from build123d import *

# Parameters (mm, degrees)
ESBO_O1_R                = 3.5
ESBO_O1_R_2              = 3
ESBO_O1_R_3              = 1.6
RESSALTO_EXTRUS_O1_DEPTH = 6


with BuildPart() as part:
    # Esboço1 → Ressalto-extrusão1 (new body)
    with BuildSketch(Plane(origin=(0, 0, 0), x_dir=(1, 0, 0), z_dir=(0, 1, 0))):
        with BuildLine():
            Line((188.965018959, -38.648697641), (188.965018959, 28))
            ThreePointArc((188.965018959, 28), (185.450300333, 36.485281374), (176.965018959, 40))
            Line((176.965018959, 40), (-176.090826953, 40))
            ThreePointArc((-176.090826953, 40), (-184.576108327, 36.485281374), (-188.090826953, 28))
            Line((-188.090826953, 28), (-188.090826953, -38.648697641))
            ThreePointArc((-188.090826953, -38.648697641), (-184.576108327, -47.133979015), (-176.090826953, -50.648697641))
            Line((-176.090826953, -50.648697641), (176.965018959, -50.648697641))
            ThreePointArc((176.965018959, -50.648697641), (185.450300333, -47.133979015), (188.965018959, -38.648697641))
        make_face()
        with Locations(Location((-62.734509176, 0, 0), (0, 0, 90))):
            Circle(ESBO_O1_R, mode=Mode.SUBTRACT)
        with Locations(Location((176.748138959, -38.431817641, 0), (0, 0, 90))):
            Circle(ESBO_O1_R_2, mode=Mode.SUBTRACT)
        with Locations(Location((0.437096003, -38.431817641, 0), (0, 0, 90))):
            Circle(ESBO_O1_R_2, mode=Mode.SUBTRACT)
        with Locations(Location((79.965018959, 10, 0), (0, 0, 90))):
            Circle(ESBO_O1_R_2, mode=Mode.SUBTRACT)
        with Locations(Location((-140.090826953, 10, 0), (0, 0, 90))):
            Circle(ESBO_O1_R, mode=Mode.SUBTRACT)
        with Locations(Location((-148.090826953, 0, 0), (0, 0, 270))):
            Circle(ESBO_O1_R_3, mode=Mode.SUBTRACT)
        with Locations(Location((-132.090826953, 0, 0), (0, 0, 270))):
            Circle(ESBO_O1_R_3, mode=Mode.SUBTRACT)
        with Locations(Location((-132.090826953, 20, 0), (0, 0, 270))):
            Circle(ESBO_O1_R_3, mode=Mode.SUBTRACT)
        with Locations(Location((-148.090826953, 20, 0), (0, 0, 270))):
            Circle(ESBO_O1_R_3, mode=Mode.SUBTRACT)
        with Locations(Location((-70.734509176, -10, 0), (0, 0, 270))):
            Circle(ESBO_O1_R_3, mode=Mode.SUBTRACT)
        with Locations(Location((-70.734509176, 10, 0), (0, 0, 270))):
            Circle(ESBO_O1_R_3, mode=Mode.SUBTRACT)
        with Locations(Location((-54.734509176, 10, 0), (0, 0, 270))):
            Circle(ESBO_O1_R_3, mode=Mode.SUBTRACT)
        with Locations(Location((-54.734509176, -10, 0), (0, 0, 270))):
            Circle(ESBO_O1_R_3, mode=Mode.SUBTRACT)
        with Locations(Location((-83.930342624, 32.5, 0), (0, 0, 90))):
            Circle(ESBO_O1_R_2, mode=Mode.SUBTRACT)
        with Locations(Location((-175.873946953, -38.431817641, 0), (0, 0, 90))):
            Circle(ESBO_O1_R_2, mode=Mode.SUBTRACT)
        with Locations(Location((140.965018959, 10, 0), (0, 0, 90))):
            Circle(ESBO_O1_R, mode=Mode.SUBTRACT)
        with Locations(Location((148.965018959, 0, 0), (0, 0, 90))):
            Circle(ESBO_O1_R_3, mode=Mode.SUBTRACT)
        with Locations(Location((148.965018959, 20, 0), (0, 0, 90))):
            Circle(ESBO_O1_R_3, mode=Mode.SUBTRACT)
        with Locations(Location((132.965018959, 0, 0), (0, 0, 90))):
            Circle(ESBO_O1_R_3, mode=Mode.SUBTRACT)
        with Locations(Location((132.965018959, 20, 0), (0, 0, 90))):
            Circle(ESBO_O1_R_3, mode=Mode.SUBTRACT)
    extrude(amount=-RESSALTO_EXTRUS_O1_DEPTH)


solid = part.part
CAD build for the part. Positions are in the model's coordinates, mm. Round coordinates to 2 decimals unless told otherwise and drop trailing zeros. Put each result on its own line as item: value.
1. Wall check: line 1 (X direction, y = -1.95, z = -20); line 2 (X direction, y = -3.6, z = 10); line 3 (Z direction, x = 133, y = -3.4). Give the ranges that are in metal, low to high.
Geometry check:
line 1: -188.09 to -149.69, -146.49 to -133.69, -130.49 to 131.37, 134.57 to 147.37, 150.57 to 188.97
line 2: -188.09 to -72.33, -69.13 to -56.33, -53.13 to 188.97
line 3: -40 to -21.6, -18.4 to -1.6, 1.6 to 50.65
2. Two-plate mould, pull along Z, no slides. Class faces 1 (the flat face through (-2, -3, 50.649)), 2 (the flat face through (-2, -6, 5)), 3 (the cylindrical face through (0.31, -2.96, 41.43)): released by +Z, released by -Z, zero draft, split by the parting line, or undercut.
Geometry check:
face 1: released by +Z
face 2: zero draft
face 3: undercut
3. Pin check, flat tips, straight feed: P1, Ø4, axis at x = -148.09, z = 0, coming from the +Y side; P2, Ø5.5, axis at x = 79.97, z = -10, coming from the +Y side. Stop position of each tip, or through.
Geometry check:
P1: y = 0
P2: through
